```python
from build123d import *

# Parameters (mm, degrees)
SKETCH1_W           = 685.8
SKETCH1_H           = 38.1
BOSS_EXTRUDE1_DEPTH = 6.35
SKETCH2_W           = 50.8
SKETCH2_H           = 25.4
BOSS_EXTRUDE2_DEPTH = 6.35
SKETCH3_W           = 7.62
SKETCH3_H           = 6.35
CUT_EXTRUDE1_DEPTH  = 7.35
SKETCH4_W           = 6.35
SKETCH4_H           = 19.05
CUT_EXTRUDE2_DEPTH  = 7.35


with BuildPart() as part:
    # Sketch1 → Boss-Extrude1 (new body)
    with BuildSketch(Plane.XY):
        Rectangle(SKETCH1_W, SKETCH1_H)
    extrude(amount=BOSS_EXTRUDE1_DEPTH)

    # Sketch2 → Boss-Extrude2 (add)
    with BuildSketch(Plane.XY.offset(6.35)):
        with Locations((-342.9, 0)):
            Rectangle(SKETCH2_W, SKETCH2_H)
    boss_extrude2 = extrude(amount=-BOSS_EXTRUDE2_DEPTH)

    # Sketch3 → Cut-Extrude1 (cut, through all)
    with BuildSketch(Plane.XY.offset(6.35)):
        with Locations((-351.79, 0)):
            Rectangle(SKETCH3_W, SKETCH3_H)
    cut_extrude1 = extrude(amount=-CUT_EXTRUDE1_DEPTH, mode=Mode.SUBTRACT)

    # Mirror1: Boss-Extrude2, Cut-Extrude1 across plane
    add(boss_extrude2.mirror(Plane(origin=(0, 0, 0), x_dir=(0, 0, 1), z_dir=(1, 0, 0))))
    add(cut_extrude1.mirror(Plane(origin=(0, 0, 0), x_dir=(0, 0, 1), z_dir=(1, 0, 0))), mode=Mode.SUBTRACT)

    # Sketch4 → Cut-Extrude2 (cut, through all)
    with BuildSketch(Plane.XY.offset(6.35)):
        with Locations((-203.2, 0)):
            Rectangle(SKETCH4_W, SKETCH4_H)
    cut_extrude2 = extrude(amount=-CUT_EXTRUDE2_DEPTH, mode=Mode.SUBTRACT)

    # Mirror2: Cut-Extrude2 across plane
    add(cut_extrude2.mirror(Plane(origin=(0, 0, 0), x_dir=(0, 0, 1), z_dir=(1, 0, 0))), mode=Mode.SUBTRACT)


solid = part.part
```
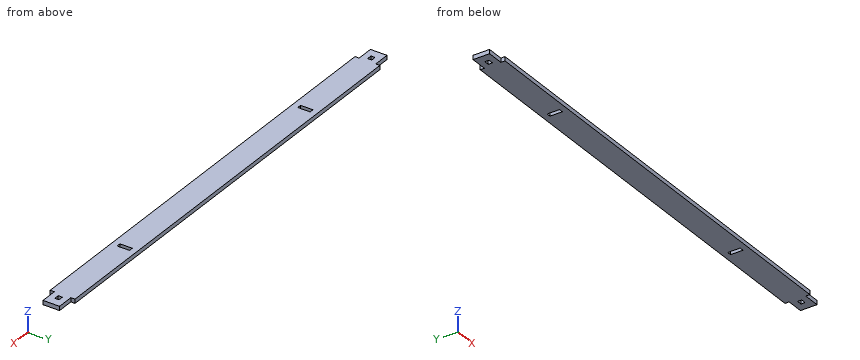
Work out the finished part from the listing and answer in its coordinate system (mm). Round coordinates to 2 decimals unless told otherwise and drop trailing zeros. Loops run counter-clockwise (first coordinate to the right, second up) from the corner with the lowest first, then second, coordinate; pieces in that order, holes last. Notation, with made-up numbers: M -12.75,82 L 12.25,82 A8 ccw 12.25,90 Z; hole C 78,41.25 d3. An arc over 180 degrees is marked long. One line per question, with ' | ' between items.
Q1. Each of these flat-tipped pins is pushed along its axis until it touches: pin 1 Ø3 at (x, z) = (352.5, 2) entering from -Y; pin 2 Ø8 at (x, y) = (-57.5, 3) entering from -Z; pin 3 Ø1.9 at (y, z) = (16.5, 4) entering from -X. Where does it stop, or does it pass through?
Conclusion:
pin 1: stops at y = -12.7 | pin 2: stops at z = 0 | pin 3: stops at x = -342.9
Q2. Find section A-A, the plane z = 2.25. Give the vertices of the cut face in (x, y) (3 decimals), then the cut area to 3 significant figures.
Conclusion:
outline: M -368.3,-12.7 L -342.9,-12.7 L -342.9,-19.05 L 342.9,-19.05 L 342.9,-12.7 L 368.3,-12.7 L 368.3,12.7 L 342.9,12.7 L 342.9,19.05 L -342.9,19.05 L -342.9,12.7 L -368.3,12.7 Z; hole M -355.6,-3.175 L -347.98,-3.175 L -347.98,3.175 L -355.6,3.175 Z; hole M -206.375,-9.525 L -200.025,-9.525 L -200.025,9.525 L -206.375,9.525 Z; hole M 200.025,-9.525 L 206.375,-9.525 L 206.375,9.525 L 200.025,9.525 Z; hole M 347.98,-3.175 L 355.6,-3.175 L 355.6,3.175 L 347.98,3.175 Z | area: 27,100 mm2
Q3. Consider line 1 along X through (y, z) = (-5.5, 1.5) (3 decimals); line 2 along X through (y, z) = (-1, 2.5) (3 decimals); line 3 along X through (y, z) = (17.5, 1). Determine where each line is inside the solid, lowest interval first. Write a range as from..to.
Conclusion:
line 1: x = -368.3..-206.375, -200.025..200.025, 206.375..368.3 | line 2: x = -368.3..-355.6, -347.98..-206.375, -200.025..200.025, 206.375..347.98, 355.6..368.3 | line 3: x = -342.9..342.9
